Part model, mm, in its own coordinate system. A direction names the side the tool comes from. Give positions to 0.01 mm unless a question says otherwise; leave off trailing zeros. Loops run counter-clockwise (first coordinate to the right, second up) from the corner with the lowest first, then second, coordinate; pieces in that order, holes last. Notation, with made-up numbers: M 46.25,4.5 L 62.25,4.5 A26 ccw 62.25,18.5 Z; hole C 63,53 d5. An arc over 180 degrees is marked long. Answer in a Markdown table with one row per item.
from build123d import *

# Parameters (mm, degrees)
BOSS_EXTRUDE1_DEPTH = 4
SKETCH3_W           = 130
SKETCH3_H           = 120
SKETCH3_W_2         = 125
SKETCH3_H_2         = 115
BOSS_EXTRUDE2_DEPTH = 10
FILLET1_R           = 5
FILLET2_R           = 10


with BuildPart() as part:
    # Sketch1 → Boss-Extrude1 (new body)
    with BuildSketch(Plane(origin=(0, 0, 0), x_dir=(1, 0, 0), z_dir=(0, 1, 0))):
        Polygon((-68, 63), (68, 63), (68, 39.979206653), (68, 10), (78, 10), (78, -10), (68, -10), (68, -63), (-68, -63), (-68, -10), (-78, -10), (-78, 10), (-68, 10), (-68, 39.979206653), align=None)
    extrude(amount=BOSS_EXTRUDE1_DEPTH)

    # Sketch3 → Boss-Extrude2 (add)
    with BuildSketch(Plane(origin=(0, 4, 0), x_dir=(1, 0, 0), z_dir=(0, 1, 0))):
        Rectangle(SKETCH3_W, SKETCH3_H)
        Rectangle(SKETCH3_W_2, SKETCH3_H_2, mode=Mode.SUBTRACT)
    extrude(amount=BOSS_EXTRUDE2_DEPTH)

    # Fillet1
    fillet1_edges = [part.edges().sort_by_distance(p)[0] for p in [
        (68, 2, 63),
        (-68, 2, 63),
        (-68, 2, -63),
        (68, 2, -63),
    ]]
    fillet(fillet1_edges, radius=FILLET1_R)

    # Fillet2
    fillet2_edges = [part.edges().sort_by_distance(p)[0] for p in [
        (78, 2, -10),
        (78, 2, 10),
        (-78, 2, 10),
        (-78, 2, -10),
    ]]
    fillet(fillet2_edges, radius=FILLET2_R - 0.0001)  # a hair under: the kernel refuses the full size


solid = part.part
(1) Pull direction X, two halves, no side cores. Call faces 5 (the face through (-68, 2, -34)), 6 (the face through (-1, 9, -57.5)), 7 (the face through (-1, 9, 60)): +X half, -X half, draft (parallel to the pull), parting line (faces both ways), or undercut.
Recorded:
| item | result |
|---|---|
| face 5 | -X half |
| face 6 | undercut |
| face 7 | draft |
(2) Saw through at B-B (y = 10.5). Write the cut outline in (x, z).
Recorded:
| item | result |
|---|---|
| outline | M -65,-60 L 65,-60 L 65,60 L -65,60 Z; hole M -62.5,-57.5 L 62.5,-57.5 L 62.5,57.5 L -62.5,57.5 Z |
(3) Drill centre lines: line 1 along X through (y, z) = (5.75, 0); line 2 along Z through (x, y) = (39.5, 8.5); line 3 along X through (y, z) = (1.5, 38). Where is each one in solid material? Low to high.
Recorded:
| item | result |
|---|---|
| line 1 | x = -65 to -62.5, 62.5 to 65 |
| line 2 | z = -60 to -57.5, 57.5 to 60 |
| line 3 | x = -68 to 68 |
(4) Saw through at D-D (x = -46.5). Write the cut outline in (y, z).
Recorded:
| item | result |
|---|---|
| outline | M 0,-63 L 4,-63 L 4,-60 L 14,-60 L 14,-57.5 L 4,-57.5 L 4,57.5 L 14,57.5 L 14,60 L 4,60 L 4,63 L 0,63 Z |
(5) Pin check, flat tips, straight feed: pin 1 Ø5 at (y, z) = (7, -5.5) entering from +X; pin 2 Ø3 at (y, z) = (8, 2) entering from -X; pin 3 Ø3 at (x, z) = (59, -37.5) entering from +Y. Stop position of each tip, or through.
Recorded:
| item | result |
|---|---|
| pin 1 | stops at x = 65 |
| pin 2 | stops at x = -65 |
| pin 3 | stops at y = 4 |
(6) Saw through at A-A (z = -45.5). Write the cut outline in (x, y).
Recorded:
| item | result |
|---|---|
| outline | M -68,0 L 68,0 L 68,4 L 65,4 L 65,14 L 62.5,14 L 62.5,4 L -62.5,4 L -62.5,14 L -65,14 L -65,4 L -68,4 Z |
(7) Which spindle directions (+Z, -Z, +X, -X, +Y, -Y) get a long thin tool onto all of the face, cutting with end or side? Do faces 1 (the face through (-1, 9, -60)), 2 (the face through (65, 9, 1)), 3 (the face through (68, 2, 34)), 4 (the face through (-65, 9, 1)). Say none if no direction does.
Recorded:
| item | result |
|---|---|
| face 1 | -Z, +X, -X, +Y |
| face 2 | +Z, -Z, +X, +Y |
| face 3 | +Z, +X, +Y, -Y |
| face 4 | +Z, -Z, -X, +Y |
